Part model, mm, in its own coordinate system. Round coordinates to 2 decimals unless told otherwise and drop trailing zeros. Write each loop counter-clockwise with the first axis right and the second up, starting at its lowest first coordinate (ties: lowest second). Pieces come first, ordered by that corner, then holes.
```python
from build123d import *

# Parameters (mm, degrees)
BOSS_EXTRUDE1_DEPTH = 3.175
SKETCH3_R           = 7.39
SKETCH3_R_2         = 1
CUT_EXTRUDE1_DEPTH  = 4.175


with BuildPart() as part:
    # Sketch2 → Boss-Extrude1 (new body)
    with BuildSketch(Plane.XY):
        Polygon((0, 120.65), (0, 127), (196.85, 127), (196.85, 120.65), (200.025, 120.65), (200.025, 6.35), (196.85, 6.35), (196.85, 0), (0, 0), (0, 6.35), (-3.175, 6.35), (-3.175, 120.65), align=None)
    extrude(amount=BOSS_EXTRUDE1_DEPTH)

    # Sketch3 → Cut-Extrude1 (cut, through all)
    with BuildSketch(Plane.XY.offset(3.175)):
        with Locations((98.425, 63.5)):
            Circle(SKETCH3_R)
        with Locations((88.545, 63.5)):
            Circle(SKETCH3_R_2)
        with Locations((108.357, 63.5)):
            Circle(SKETCH3_R_2)
    extrude(amount=-CUT_EXTRUDE1_DEPTH, mode=Mode.SUBTRACT)


solid = part.part
```
Q1. Wall check: L1, parallel to Y at x = 96.5, z = 0.65; L2, parallel to X at y = 121.5, z = 2.45; L3, parallel to X at y = 67, z = 0.55 (3 decimals). Give the ranges that are in metal, low to high.
Values follow:
L1: y = 0 to 56.37, 70.63 to 127
L2: x = 0 to 196.85
L3: x = -3.175 to 91.916, 104.934 to 200.025
Q2. Mould opens along Y. For faces 1 (the flat face through (100, 79, 3.175)), 2 (the cylindrical face through (105.25, 60.67, 1.61)) say: +Y half, -Y half, draft (parallel to the pull), parting line (faces both ways), or undercut.
Values follow:
face 1: draft
face 2: undercut
Q3. Cut at A-A on x = 94. Write the cut outline in (y, z) (3 decimals), plus the area to 3 significant figures.
Values follow:
outline: (0, 0) - (57.581, 0) - (57.581, 3.175) - (0, 3.175) - close; (69.419, 0) - (127, 0) - (127, 3.175) - (69.419, 3.175) - close
area: 366 mm2
Q4. Drop flat-ended pins along their axis: pin 1 (1.5 mm diameter, centred on x = 91.5, y = 109, fed in from -Z); pin 2 (1 mm diameter, centred on y = 125, z = 2, fed in from -X); pin 3 (1.6 mm diameter, centred on y = 3.5, z = 1, fed in from +X); pin 4 (1.6 mm diameter, centred on x = -2, z = 2, fed in from -Y). Give the stop position or say it passes through.
Values follow:
pin 1: stops at z = 0
pin 2: stops at x = 0
pin 3: stops at x = 196.85
pin 4: stops at y = 6.35
